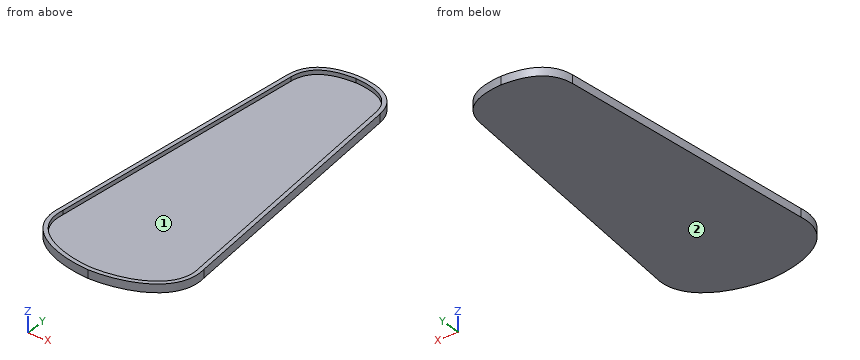
```python
from build123d import *

# Parameters (mm, degrees)
BOSS_EXTRUDE1_DEPTH = 19.05
CUT_EXTRUDE1_DEPTH  = 9.525


with BuildPart() as part:
    # Sketch2 → Boss-Extrude1 (new body)
    with BuildSketch(Plane.XY):
        with BuildLine():
            Line((-166.6875, 130.175), (-106.876080835, 736.833680097))
            add(Edge.make_bspline(
                [(-106.876080835, 736.833680097), (-98.655564568, 809.385111394), (0, 812.8)],
                knots=[0, 0, 0, 1, 1, 1], degree=2))
            add(Edge.make_bspline(
                [(106.876080835, 736.833680097), (98.655564568, 809.385111394), (0, 812.8)],
                knots=[0, 0, 0, 1, 1, 1], degree=2))
            Line((106.876080835, 736.833680097), (166.6875, 130.175))
            add(Edge.make_bspline(
                [(0, 0), (73.666580622, 1.740675992), (181.188092361, 36.200835609), (166.6875, 130.175)],
                knots=[0, 0, 0, 0, 1, 1, 1, 1], degree=3))
            add(Edge.make_bspline(
                [(0, 0), (-73.666580622, 1.740675992), (-181.188092361, 36.200835609), (-166.6875, 130.175)],
                knots=[0, 0, 0, 0, 1, 1, 1, 1], degree=3))
        make_face()
    extrude(amount=BOSS_EXTRUDE1_DEPTH)

    # Sketch4 → Cut-Extrude1 (cut)
    with BuildSketch(Plane.XY.offset(19.05)):
        with BuildLine():
            Line((-97.403993572, 735.828587026), (-157.234081882, 128.980548454))
            add(Edge.make_bspline(
                [(-157.234081882, 128.980548454), (-157.324205492, 128.396483281), (-157.412089483, 127.812410477), (-157.576084777, 126.644224751), (-157.653279282, 126.06011552), (-157.870174292, 124.307737773), (-157.995189913, 123.139419215), (-158.309135667, 119.634255327), (-158.437031706, 117.29720201), (-158.555423917, 110.285138008), (-158.282055898, 105.60922815), (-157.411253292, 99.762537833), (-157.210017909, 98.591234632), (-156.757264158, 96.273926752), (-156.001688417, 92.827229864), (-155.017022207, 89.468234028), (-152.743005414, 82.866882475), (-150.82076111, 78.621496729), (-147.913058291, 73.508050792), (-147.306271331, 72.4950265), (-146.042259928, 70.488286534), (-145.389757898, 69.50206831), (-143.374427295, 66.59388241), (-141.953452439, 64.721702461), (-137.477795564, 59.288190671), (-134.211225834, 55.909160224), (-129.824716649, 51.946319201), (-128.932947118, 51.167642375), (-127.132093683, 49.645344246), (-126.221588539, 48.900422844), (-123.461599805, 46.711504594), (-121.583697089, 45.313266475), (-115.848105381, 41.282598746), (-111.889088448, 38.81332115), (-103.746143975, 34.236903166), (-99.561981891, 32.130140428), (-94.209825099, 29.693050126), (-93.132197949, 29.215042748), (-90.971456085, 28.280905266), (-89.888342715, 27.824742202), (-86.631139254, 26.48752268), (-84.44919675, 25.6376924), (-77.874418426, 23.203328361), (-73.452755763, 21.733428424), (-64.541987933, 19.061822744), (-60.052845479, 17.860265278), (-51.012964961, 15.702093584), (-46.462212797, 14.745535421), (-37.302169602, 13.065206786), (-32.692883998, 12.341414728), (-25.735345382, 11.429148513), (-23.408876198, 11.154048031), (-18.7411174, 10.662782498), (-16.401859715, 10.446870289), (-9.382680965, 9.891490593), (-4.695544036, 9.643012505), (0, 9.52776174)],
                knots=[0, 0, 0, 0, 0.0078125, 0.0078125, 0.015625, 0.015625, 0.03125, 0.03125, 0.0625, 0.0625, 0.125, 0.125, 0.140625, 0.140625, 0.15625, 0.1875, 0.1875, 0.25, 0.25, 0.265625, 0.265625, 0.28125, 0.28125, 0.3125, 0.3125, 0.375, 0.375, 0.390625, 0.390625, 0.40625, 0.40625, 0.4375, 0.4375, 0.5, 0.5, 0.5625, 0.5625, 0.578125, 0.578125, 0.59375, 0.59375, 0.625, 0.625, 0.6875, 0.6875, 0.75, 0.75, 0.8125, 0.8125, 0.875, 0.875, 0.90625, 0.90625, 0.9375, 0.9375, 1, 1, 1, 1], degree=3))
            add(Edge.make_bspline(
                [(0, 9.52776174), (4.696782429, 9.643042901), (9.371788605, 9.891241348), (18.682630774, 10.626724118), (23.318416438, 11.114315633), (32.552071373, 12.320931698), (37.149923971, 13.040058014), (46.306955275, 14.714367272), (50.866134292, 15.669548315), (59.943247261, 17.831660883), (64.461195673, 19.038504147), (71.20372728, 21.058683944), (73.447300549, 21.767866857), (77.898983356, 23.253348365), (80.109631224, 24.030343068), (86.693442252, 26.469842463), (91.018725741, 28.240292259), (99.522601409, 32.111908605), (103.70134125, 34.212742248), (108.81530232, 37.085571172), (109.832590209, 37.672546502), (111.855568511, 38.872643767), (112.862320589, 39.486453403), (115.852002601, 41.361553617), (117.806717627, 42.657699597), (123.546532273, 46.69530685), (127.208159374, 49.584908122), (132.403942543, 54.275234083), (134.0862339, 55.898228847), (136.526821296, 58.432122427), (137.326523938, 59.293342382), (138.896628692, 61.050936516), (139.668584954, 61.949275112), (143.422485376, 66.499587265), (146.099261927, 70.337793886), (149.575356296, 76.4220986), (150.644084323, 78.504775138), (152.10493938, 81.715069485), (152.568177575, 82.799551968), (153.44592623, 84.998074695), (153.858285185, 86.106992021), (155.77907965, 91.670668847), (156.87633236, 96.211033443), (157.917859106, 103.144578031), (158.164237879, 105.476273711), (158.388791016, 109.003330668), (158.439487754, 110.186052077), (158.493329725, 112.548388418), (158.496596004, 113.728050186), (158.438962094, 117.262741174), (158.31071539, 119.613481568), (157.996011579, 123.131801583), (157.87069881, 124.303275057), (157.58107101, 126.643738225), (157.414305379, 127.812571858), (157.234081882, 128.980548454)],
                knots=[0, 0, 0, 0, 0.0625, 0.0625, 0.125, 0.125, 0.1875, 0.1875, 0.25, 0.25, 0.3125, 0.3125, 0.34375, 0.34375, 0.375, 0.375, 0.4375, 0.4375, 0.5, 0.5, 0.515625, 0.515625, 0.53125, 0.53125, 0.5625, 0.5625, 0.625, 0.625, 0.65625, 0.65625, 0.671875, 0.671875, 0.6875, 0.6875, 0.75, 0.75, 0.78125, 0.78125, 0.796875, 0.796875, 0.8125, 0.8125, 0.875, 0.875, 0.90625, 0.90625, 0.921875, 0.921875, 0.9375, 0.9375, 0.96875, 0.96875, 0.984375, 0.984375, 1, 1, 1, 1], degree=3))
            Line((157.234081882, 128.980548454), (97.403993572, 735.828587022))
            add(Edge.make_bspline(
                [(97.403993572, 735.828587022), (97.092286958, 738.562982934), (96.669418738, 741.267379451), (95.570059645, 746.607726854), (94.893642768, 749.243697709), (93.247932944, 754.436600394), (92.278730315, 756.993556598), (90.853060681, 760.13195437), (90.557097177, 760.756799005), (89.94756396, 761.991267361), (89.633481965, 762.602053668), (88.66308079, 764.414924295), (87.978602457, 765.597517573), (85.810987946, 769.066265293), (84.213589669, 771.273330454), (81.584120863, 774.422394534), (80.668756062, 775.44517415), (79.236968861, 776.938685261), (78.749736274, 777.429849509), (77.763144525, 778.391567332), (77.262906247, 778.863062984), (72.700160744, 783.024790933), (68.215938322, 786.146253506), (62.187228676, 789.476997053), (60.964200371, 790.112025219), (58.502000457, 791.317342862), (57.260396611, 791.888985895), (53.506907039, 793.519234755), (50.966447444, 794.493467918), (43.248745942, 797.131746553), (37.976068957, 798.513992185), (31.266175529, 799.890277732), (29.917456906, 800.147831744), (27.218689157, 800.627892818), (25.867458716, 800.850662293), (21.808637288, 801.471016253), (19.095929317, 801.820768942), (10.940039087, 802.703953619), (5.479213552, 803.072462364), (2e-09, 803.26908628)],
                knots=[0, 0, 0, 0, 0.0625, 0.0625, 0.125, 0.125, 0.1875, 0.1875, 0.203125, 0.203125, 0.21875, 0.21875, 0.25, 0.25, 0.3125, 0.3125, 0.34375, 0.34375, 0.359375, 0.359375, 0.375, 0.375, 0.5, 0.5, 0.53125, 0.53125, 0.5625, 0.5625, 0.625, 0.625, 0.75, 0.75, 0.78125, 0.78125, 0.8125, 0.8125, 0.875, 0.875, 1, 1, 1, 1], degree=3))
            add(Edge.make_bspline(
                [(2e-09, 803.26908628), (-5.471123606, 803.072752675), (-10.913888363, 802.705230434), (-21.727709567, 801.537317666), (-27.098938668, 800.737969365), (-35.084786769, 799.110381206), (-37.734826452, 798.495958833), (-43.006804741, 797.097481507), (-45.628764384, 796.313553549), (-49.536321772, 794.984442323), (-50.832509452, 794.516370139), (-53.395578467, 793.531913824), (-54.664623053, 793.014810614), (-58.431517441, 791.383359846), (-60.889276194, 790.189166552), (-65.679911837, 787.552063988), (-68.012848984, 786.109274725), (-72.530602319, 782.928697006), (-74.672229275, 781.220279014), (-78.696640654, 777.560904851), (-80.581086505, 775.608725668), (-83.205841084, 772.486867934), (-84.047113279, 771.413989968), (-85.660763906, 769.202180872), (-86.433815235, 768.062175102), (-90.116138831, 762.204478677), (-92.353845254, 757.218061553), (-94.440219005, 750.683674858), (-94.821772855, 749.361651688), (-95.517065206, 746.688851322), (-95.829087041, 745.344622952), (-96.665508178, 741.295731389), (-97.091208587, 738.572442767), (-97.403993572, 735.828587026)],
                knots=[0, 0, 0, 0, 0.125, 0.125, 0.25, 0.25, 0.3125, 0.3125, 0.375, 0.375, 0.40625, 0.40625, 0.4375, 0.4375, 0.5, 0.5, 0.5625, 0.5625, 0.625, 0.625, 0.6875, 0.6875, 0.71875, 0.71875, 0.75, 0.75, 0.875, 0.875, 0.90625, 0.90625, 0.9375, 0.9375, 1, 1, 1, 1], degree=3))
        make_face()
    extrude(amount=-CUT_EXTRUDE1_DEPTH, mode=Mode.SUBTRACT)


solid = part.part
```
Work out the finished part from the listing and answer in its coordinate system (mm). Face numbers are marked on the shaded views. Coordinates: 2 decimals unless noted, no trailing zeros. Write each loop counter-clockwise with the first axis right and the second up, starting at its lowest first coordinate (ties: lowest second). Pieces come first, ordered by that corner, then holes.
Q1. A cutting plane is placed at A-A, the plane y = 179.5. Give the vertices of the cut face in (x, z) (3 decimals).
Q2. Determine the mould class of the marked faces 1 and 2 for opening direction X: released by +X, released by -X, zero draft, split by the parting line, or undercut.
Q3. Find the intervals of material crossed by line 1 (Z direction, x = -57.5, y = 404.5) (3 decimals); line 2 (X direction, y = 572, z = 12); line 3 (X direction, y = 621, z = 16.5), in increasing order.
Q4. A cutting plane is placed at B-B, the plane y = 581.5. Give the vertices of the cut face in (x, z) (3 decimals), then the cut area to 3 significant figures.
Q5. Each of these flat-tipped pins is pushed along its axis until it touches: pin 1 Ø1.5 at (y, z) = (483.5, 10) entering from +X; pin 2 Ø3 at (x, z) = (-83.5, 12.5) entering from -Y; pin 3 Ø1 at (x, y) = (-6.5, 368.5) entering from +Z (3 decimals). Where does it stop, or does it pass through?
Findings below:
1. outline: (-161.824, 0) - (161.824, 0) - (161.824, 19.05) - (152.253, 19.05) - (152.253, 9.525) - (-152.253, 9.525) - (-152.253, 19.05) - (-161.824, 19.05) - close
2. face 1: undercut
2. face 2: zero draft
3. line 1: z = 0 to 9.525
3. line 2: x = -123.13 to -113.56, 113.56 to 123.13
3. line 3: x = -118.3 to -108.73, 108.73 to 118.3
4. outline: (-122.191, 0) - (122.191, 0) - (122.191, 19.05) - (112.619, 19.05) - (112.619, 9.525) - (-112.619, 9.525) - (-112.619, 19.05) - (-122.191, 19.05) - close
4. area: 2,510 mm2
5. pin 1: stops at x = 131.93
5. pin 2: stops at y = 14.61
5. pin 3: stops at z = 9.525
